Read the model definition and answer for the solid it produces. Units are mm, in the model's axes. Face numbers are marked on the shaded views. Coordinates: 2 decimals unless noted, no trailing zeros. Order: outer loops, then holes, each group sorted by start corner. A loop starts at its lowest first (then second) coordinate and runs counter-clockwise, first axis right, second up.
```python
from build123d import *

# Parameters (mm, degrees)
SKETCH1_W           = 58.42
SKETCH1_H           = 96.52
SKETCH1_W_2         = 52.07
SKETCH1_H_2         = 90.17
BOSS_EXTRUDE1_DEPTH = 6.35
SKETCH1_4_W         = 58.42
SKETCH1_4_H         = 96.52
BOSS_EXTRUDE2_DEPTH = 3.175
FILLET1_R           = 6.35
SKETCH4_W           = 52.07
SKETCH4_H           = 20.225419923
CUT_EXTRUDE2_DEPTH  = 6.35
SKETCH5_W           = 78.910757724
SKETCH5_H           = 12.7
CUT_EXTRUDE3_DEPTH  = 6.35
FILLET2_R           = 1.5875
FILLET3_R           = 7.9375
CHAMFER2_SIZE       = 0.635


with BuildPart() as part:
    # Sketch1 → Boss-Extrude1 (new body)
    with BuildSketch(Plane(origin=(0, 0, 0), x_dir=(1, 0, 0), z_dir=(0, 1, 0))):
        Rectangle(SKETCH1_W, SKETCH1_H)
        Rectangle(SKETCH1_W_2, SKETCH1_H_2, mode=Mode.SUBTRACT)
    extrude(amount=BOSS_EXTRUDE1_DEPTH)

    # Sketch1<4> → Boss-Extrude2 (add)
    with BuildSketch(Plane(origin=(0, 0, 0), x_dir=(1, 0, 0), z_dir=(0, 1, 0))):
        Rectangle(SKETCH1_4_W, SKETCH1_4_H)
    extrude(amount=-BOSS_EXTRUDE2_DEPTH)

    # Fillet1
    fillet1_edges = [part.edges().sort_by_distance(p)[0] for p in [
        (26.035, 3.175, 45.085),
        (26.035, 3.175, -45.085),
        (-26.035, 3.175, -45.085),
        (-26.035, 3.175, 45.085),
    ]]
    fillet(fillet1_edges, radius=FILLET1_R)

    # Sketch4 → Cut-Extrude2 (cut)
    with BuildSketch(Plane(origin=(0, 6.35, 0), x_dir=(1, 0, 0), z_dir=(0, 1, 0))):
        with Locations((0, 43.394544924)):
            Rectangle(SKETCH4_W, SKETCH4_H)
    extrude(amount=-CUT_EXTRUDE2_DEPTH, mode=Mode.SUBTRACT)

    # Sketch5 → Cut-Extrude3 (cut)
    with BuildSketch(Plane(origin=(0, 6.35, 0), x_dir=(1, 0, 0), z_dir=(0, 1, 0))):
        Rectangle(SKETCH5_W, SKETCH5_H)
    extrude(amount=-CUT_EXTRUDE3_DEPTH, mode=Mode.SUBTRACT)

    # Fillet2
    fillet2_edges = [part.edges().sort_by_distance(p)[0] for p in [
        (29.21, 3.175, -6.35),
        (-29.21, 3.175, -6.35),
        (26.035, 3.175, -6.35),
        (-26.035, 3.175, -6.35),
        (29.21, 3.175, 6.35),
        (-29.21, 3.175, 6.35),
        (26.035, 3.175, 6.35),
        (-26.035, 3.175, 6.35),
        (-29.21, 1.5875, -48.26),
        (29.21, 1.5875, -48.26),
        (26.035, 3.175, -48.26),
        (-26.035, 3.175, -48.26),
    ]]
    fillet(fillet2_edges, radius=FILLET2_R - 0.0001)  # a hair under: the kernel refuses the full size

    # Fillet3
    fillet3_edges = [part.edges().sort_by_distance(p)[0] for p in [
        (-29.21, 1.5875, 48.26),
        (29.21, 1.5875, 48.26),
    ]]
    fillet(fillet3_edges, radius=FILLET3_R)

    # Chamfer2
    chamfer2_edges = [part.edges().sort_by_distance(p)[0] for p in [
        (29.21, 6.35, -27.305),
        (-29.21, 6.35, 24.12995),
        (-26.035, 6.35, 23.3362),
        (-28.745061304, 6.35, 6.814938696),
        (-26.499938696, 6.35, 6.814938696),
        (26.499938696, 6.35, 6.814938696),
        (28.745061304, 6.35, 6.814938696),
        (26.035, 6.35, -27.305),
        (26.499938696, 6.35, -47.795061304),
        (28.745061304, 6.35, -47.795061304),
        (26.499938696, 6.35, -6.814938696),
        (28.745061304, 6.35, -6.814938696),
        (-29.21, 6.35, -27.305),
        (-26.035, 6.35, -27.305),
        (-26.499938696, 6.35, -47.795061304),
        (-28.745061304, 6.35, -47.795061304),
        (-28.745061304, 6.35, -6.814938696),
        (-26.499938696, 6.35, -6.814938696),
        (0, -3.175, -48.26),
        (-28.745061304, -3.175, -47.795061304),
        (28.745061304, -3.175, -47.795061304),
        (29.21, 6.35, 24.12995),
        (29.21, -3.175, -3.17505),
        (0, -3.175, 48.26),
        (-29.21, -3.175, -3.17505),
        (-26.885160076, -3.175, 45.935160076),
        (26.885160076, -3.175, 45.935160076),
        (0, 6.35, 48.26),
        (-26.885160076, 6.35, 45.935160076),
        (26.885160076, 6.35, 45.935160076),
        (26.035, 6.35, 23.3362),
        (0, 6.35, 45.085),
        (24.175128061, 6.35, 43.225128061),
        (-24.175128061, 6.35, 43.225128061),
    ]]
    chamfer(chamfer2_edges, length=CHAMFER2_SIZE)


solid = part.part
```
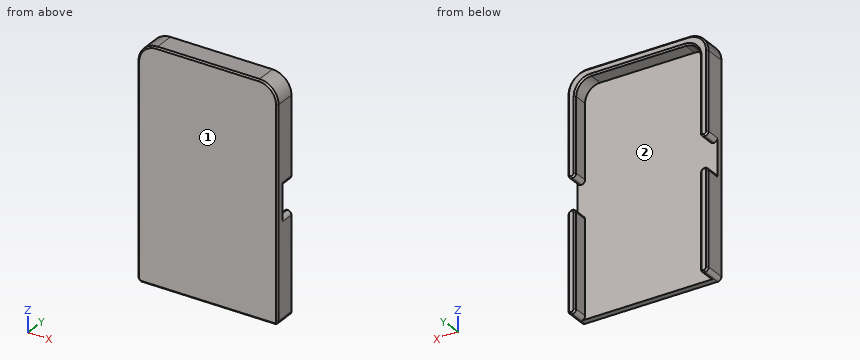
1) A cutting plane is placed at C-C, the plane z = -9. Determine the outline of the cut face in (x, y) (3 decimals), and give its area (3 significant figures).
A:
outline: (-29.21, -2.54) - (-28.575, -3.175) - (28.575, -3.175) - (29.21, -2.54) - (29.21, 5.715) - (28.575, 6.35) - (26.67, 6.35) - (26.035, 5.715) - (26.035, 0) - (-26.035, 0) - (-26.035, 5.715) - (-26.67, 6.35) - (-28.575, 6.35) - (-29.21, 5.715) - close
area: 225 mm2
2) A cutting plane is placed at A-A, the plane y = 4.75. State how many separate pieces and enclosed holes the cut face has, and give its area (3 significant figures).
A:
separate pieces: 3
enclosed holes: 0
area: 681 mm2
3) Straight lines are drawn through the part: line 1 (X direction, y = 2.5, z = 27) (3 decimals); line 2 (Y direction, x = 15.5, z = 32.5) (3 decimals); line 3 (Z direction, x = -17, y = 0.5) (3 decimals). For each, find the intervals that lie inside material, in ascending order.
A:
line 1: x = -29.21 to -26.035, 26.035 to 29.21
line 2: y = -3.175 to 0
line 3: z = 45.085 to 48.26
4) A cutting plane is placed at D-D, the plane z = 4.5. Determine the outline of the cut face in (x, y) (3 decimals).
A:
outline: (-29.21, -2.54) - (-28.575, -3.175) - (28.575, -3.175) - (29.21, -2.54) - (29.21, 0) - (-29.21, 0) - close
5) Flat-ended cylindrical pins translate along their axes: pin 1 Ø1 at (x, z) = (5.5, -30.5) entering from +Y; pin 2 Ø1.7 at (x, y) = (5, 2.5) entering from -Z (3 decimals). Find the tip coordinate at first contact, or state that the pin passes through.
A:
pin 1: stops at y = 0
pin 2: stops at z = 45.085
6) Determine the mould class of the marked faces 1 and 2 for opening direction X: pulls with the +X half, pulls with the -X half, needs draft (parallel to the pull), parting line crosses it, or undercut.
A:
face 1: needs draft
face 2: undercut
7) A cutting plane is placed at B-B, the plane x = 7. Determine the outline of the cut face in (y, z) (3 decimals), and give its area (3 significant figures).
A:
outline: (-3.175, -47.625) - (-2.54, -48.26) - (0, -48.26) - (0, 45.085) - (5.715, 45.085) - (6.35, 45.72) - (6.35, 47.625) - (5.715, 48.26) - (-2.54, 48.26) - (-3.175, 47.625) - close
area: 326 mm2
